The figure shows three views and two pictorial views of one solid part (mm, origin at its lowest corner). Answer the questions. A direction names the side the tool comes from. Coordinates: 2 decimals unless noted, no trailing zeros. Order: outer loops, then holes, each group sorted by start corner. A loop starts at its lowest first (then second) coordinate and runs counter-clockwise, first axis right, second up.
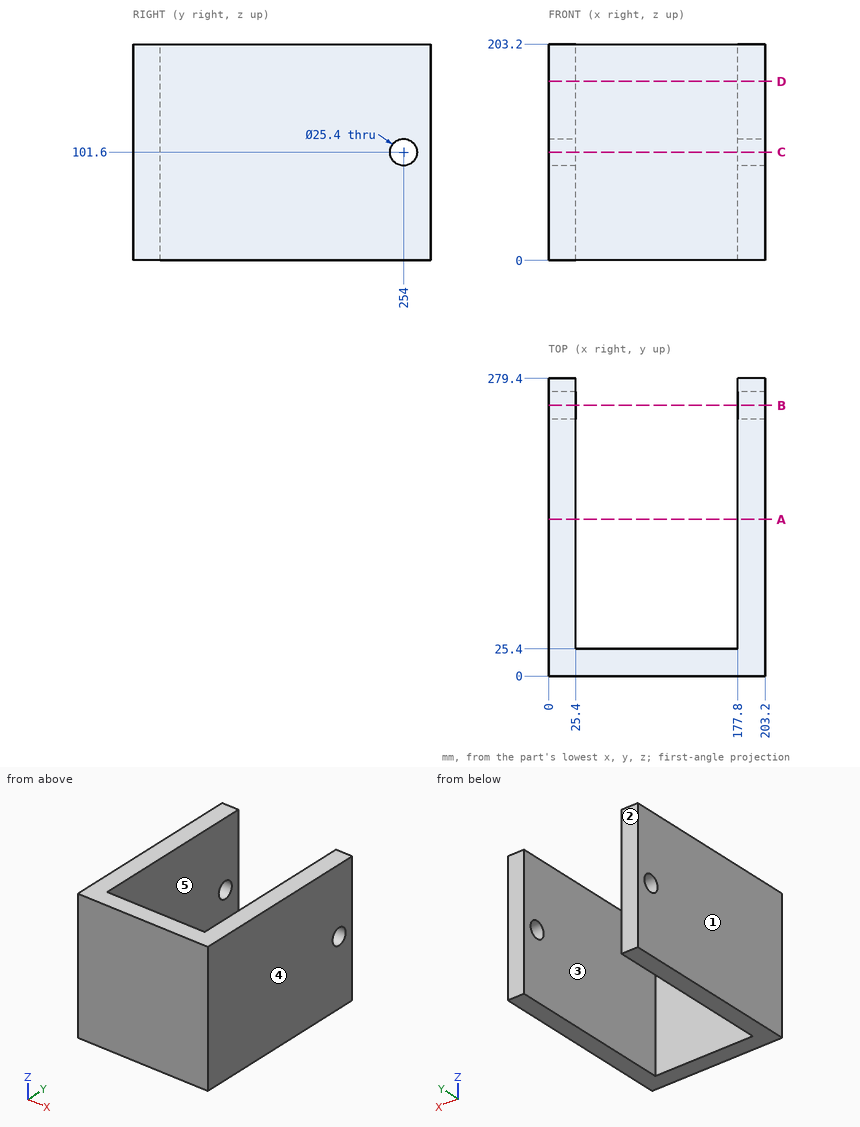
Q1. The part is cut by section A-A, the plane y = 147. Determine the outline of the cut face in (x, z), then the cut area to 3 significant figures.
Q2. Determine the mould class of the marked faces 1, 2 and 3 for opening direction X: +X half, -X half, draft (parallel to the pull), parting line (faces both ways), or undercut.
Q3. The part is cut by section D-D, the plane z = 168. Determine the outline of the cut face in (x, y).
Q4. The part is cut by section C-C, the plane z = 101.6. Determine the outline of the cut face in (x, y), then the cut area to 3 significant figures.
Q5. Straight lines are drawn through the part: L1, parallel to X at y = 131, z = 51; L2, parallel to Y at x = 184, z = 101; L3, parallel to Y at x = 85, z = 171. For each, find the intervals that lie inside material, in ascending order.
Q6. Each of these flat-tipped pins is pushed along its axis until it touches: P1, Ø12, axis at x = 112.5, z = 28.5, coming from the +Y side; P2, Ø8, axis at y = 238.5, z = 110.5, coming from the -X side; P3, Ø23, axis at y = 254, z = 101.6, coming from the +X side. Where does it stop, or does it pass through?
Q7. Which of the six approach directions +Z, -Z, +X, -X, +Y, -Y give full straight-line access (tool end or side, diameter ignored) to the marked faces 4 and 5?
Q8. The part is cut by section B-B, the plane y = 254. Determine the outline of the cut face in (x, z), then the cut area to 3 significant figures.
Computed values:
1. outline: (0, 0) - (25.4, 0) - (25.4, 203.2) - (0, 203.2) - close; (177.8, 0) - (203.2, 0) - (203.2, 203.2) - (177.8, 203.2) - close
1. area: 10,300 mm2
2. face 1: -X half
2. face 2: draft
2. face 3: undercut
3. outline: (0, 0) - (203.2, 0) - (203.2, 279.4) - (177.8, 279.4) - (177.8, 25.4) - (25.4, 25.4) - (25.4, 279.4) - (0, 279.4) - close
4. outline: (0, 0) - (203.2, 0) - (203.2, 241.3) - (177.8, 241.3) - (177.8, 25.4) - (25.4, 25.4) - (25.4, 241.3) - (0, 241.3) - close; (0, 266.7) - (25.4, 266.7) - (25.4, 279.4) - (0, 279.4) - close; (177.8, 266.7) - (203.2, 266.7) - (203.2, 279.4) - (177.8, 279.4) - close
4. area: 16,800 mm2
5. L1: x = 0 to 25.4, 177.8 to 203.2
5. L2: y = 0 to 241.31, 266.69 to 279.4
5. L3: y = 0 to 25.4
6. P1: stops at y = 25.4
6. P2: stops at x = 0
6. P3: passes through
7. face 4: +Z, -Z, +X, +Y, -Y
7. face 5: +Z, -Z, +Y
8. outline: (0, 0) - (25.4, 0) - (25.4, 88.9) - (0, 88.9) - close; (0, 114.3) - (25.4, 114.3) - (25.4, 203.2) - (0, 203.2) - close; (177.8, 0) - (203.2, 0) - (203.2, 88.9) - (177.8, 88.9) - close; (177.8, 114.3) - (203.2, 114.3) - (203.2, 203.2) - (177.8, 203.2) - close
8. area: 9,030 mm2
